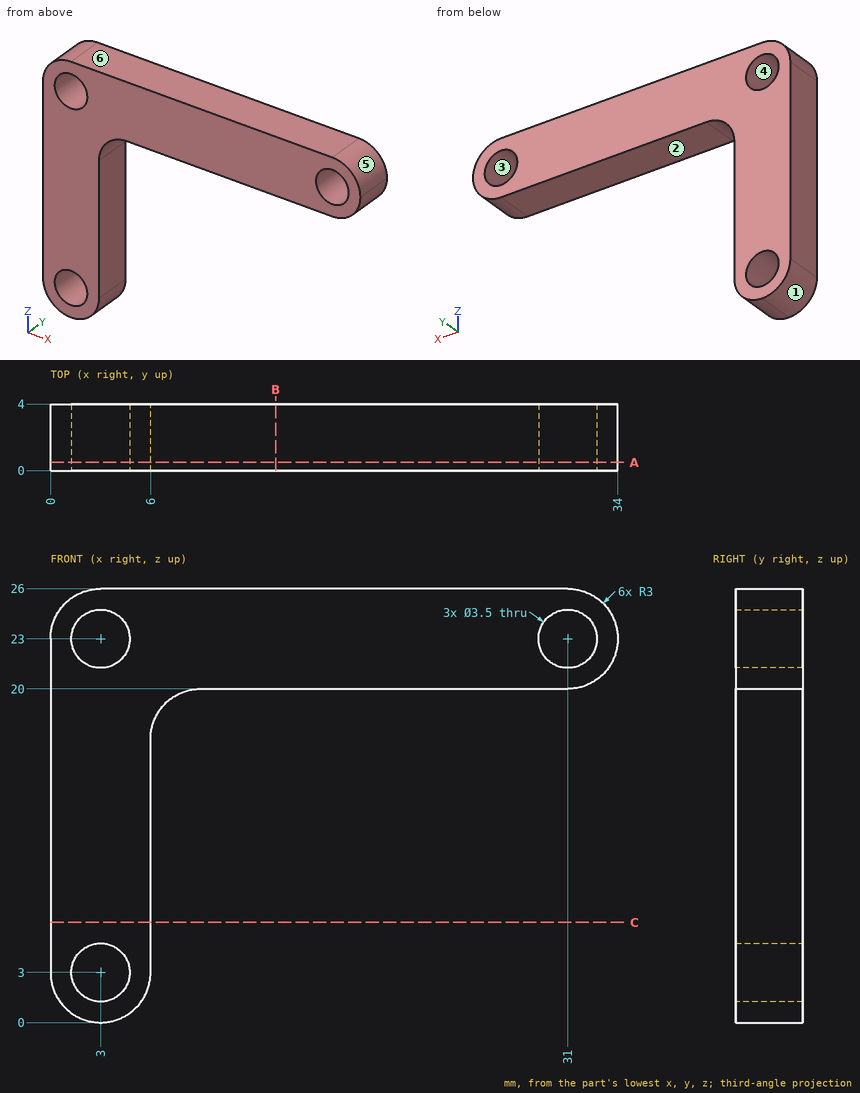
Source: three-view drawing plus pictorial views. Frame: mm from the lowest corner of the part. A direction names the side the tool comes from. Coordinates: 2 decimals unless noted, no trailing zeros. Loops run counter-clockwise (first coordinate to the right, second up) from the corner with the lowest first, then second, coordinate; pieces in that order, holes last. Notation, with made-up numbers: (-36.5, 43) -> (-21.5, 43) arc R33 ccw to (-21.5, 78) -> close; hole circle Ø8 at (2, -34.75). An arc over 180 degrees is marked (long way). Answer in a Markdown table with one row per item. Add a question column.
Q1. Section B-B on x = 13.5. Return the cut outline in (y, z).
Q2. Section A-A on y = 0.5. Give the number of separate pieces and of enclosed holes in the cut face, and give its area (3 significant figures).
Q3. Ray query, line 1 along X through (y, z) = (2.1, 23); line 2 along X through (y, z) = (1.2, 3); line 3 along Z through (x, y) = (4.5, 3). Return the intervals inside material, ascending.
Q4. Section C-C on z = 6. Return the cut outline in (x, y).
Q5. Pull-direction query (X, two-part tool) for the marked faces 3, 4, 5 and 6; classes: pulls with the +X half, pulls with the -X half, needs draft (parallel to the pull), parting line crosses it, or undercut.
Q6. Reachability of the marked faces 1 and 2 from +Z, -Z, +X, -X, +Y, -Y: full face, straight path, thin tool, end or side. Return the list, or none.
Computed values:
| question | item | result |
|---|---|---|
| 1 | outline | (0, 20) -> (4, 20) -> (4, 26) -> (0, 26) -> close |
| 2 | separate pieces | 1 |
| 2 | enclosed holes | 3 |
| 2 | area | 287 mm^2 |
| 3 | line 1 | x = 0 to 1.25, 4.75 to 29.25, 32.75 to 34 |
| 3 | line 2 | x = 0 to 1.25, 4.75 to 6 |
| 3 | line 3 | z = 0.4 to 2.1, 3.9 to 22.1, 23.9 to 26 |
| 4 | outline | (0, 0) -> (6, 0) -> (6, 4) -> (0, 4) -> close |
| 5 | face 3 | undercut |
| 5 | face 4 | undercut |
| 5 | face 5 | pulls with the +X half |
| 5 | face 6 | needs draft |
| 6 | face 1 | -Z, -X, +Y, -Y |
| 6 | face 2 | -Z, +X, +Y, -Y |
